Geometry: final body of the model. Coordinates: model frame, mm. Round coordinates to 2 decimals unless told otherwise and drop trailing zeros. Loops run counter-clockwise (first coordinate to the right, second up) from the corner with the lowest first, then second, coordinate; pieces in that order, holes last. Notation, with made-up numbers: M 41,-34 L 90,-34 A18 ccw 90,-30 Z; hole C 85.5,-13.75 d1. An arc over 180 degrees is marked long. Write each question's results on one line, items separated by ' | '.
```python
from build123d import *

# Parameters (mm, degrees)
EXTRUDE_1_DEPTH   = 2
HOLE_WIZARD_M81_D = 9
CHAMFER_1_SIZE    = 2.5


with BuildPart() as part:
    # Эскиз3 → Бобышка-Вытянуть1 (new body)
    with BuildSketch(Plane(origin=(0, 0, 0), x_dir=(1, 0, 0), z_dir=(0, 0, -1))):
        Polygon((0, 0), (100, 0), (100, 75.031110223), (87.059047745, 123.327401537), (0, 100), align=None)
    extrude(amount=EXTRUDE_1_DEPTH)

    # Отверстие с зазором M81 (through all)
    with Locations(Plane(origin=(0, 0, -2), x_dir=(1, 0, 0), z_dir=(0, 0, -1))):
        with Locations((75, 25), (24.776246401, 80.756870704), (69.381378215, 92.708779752), (25, 25)):
            Hole(HOLE_WIZARD_M81_D / 2)

    # Фаска1
    chamfer_1_edges = [part.edges().sort_by_distance(p)[0] for p in [
        (87.059047745, -123.327401537, -1),
        (100, 0, -1),
        (0, 0, -1),
    ]]
    chamfer(chamfer_1_edges, length=CHAMFER_1_SIZE)


solid = part.part
```
1. Pin query (flat end, axial travel): P1, Ø7, axis at x = 24.78, y = -80.76, coming from the -Z side. Return the tip coordinate at first contact, or that it passes through.
Answer key:
P1: passes through
2. Section B-B (x = 26). Output: boundary loops of the cut face in (y, z), then the cut area to 3 significant figures.
Answer key:
outline: M -106.97,-2 L -85.09,-2 L -85.09,0 L -106.97,0 Z; M -76.43,-2 L -29.39,-2 L -29.39,0 L -76.43,0 Z; M -20.61,-2 L 0,-2 L 0,0 L -20.61,0 Z | area: 179 mm²
3. Section C-C (y = -83.5). Output: boundary loops of the cut face in (x, z), then the cut area to 3 significant figures.
Answer key:
outline: M 0,-2 L 21.21,-2 L 21.21,0 L 0,0 Z; M 28.34,-2 L 97.73,-2 L 97.73,0 L 28.34,0 Z | area: 181 mm²
4. Section D-D (z = -0.35). Output: boundary loops of the cut face in (x, y).
Answer key:
outline: M 0,-100 L 84.64,-122.68 L 87.71,-120.91 L 100,-75.03 L 100,-2.5 L 97.5,0 L 2.5,0 L 0,-2.5 Z; hole C 24.78,-80.76 d9; hole C 25,-25 d9; hole C 69.38,-92.71 d9; hole C 75,-25 d9
5. Section A-A (y = -25). Output: boundary loops of the cut face in (x, z).
Answer key:
outline: M 0,-2 L 20.5,-2 L 20.5,0 L 0,0 Z; M 29.5,-2 L 70.5,-2 L 70.5,0 L 29.5,0 Z; M 79.5,-2 L 100,-2 L 100,0 L 79.5,0 Z
6. Draft query along X for faces 1 (the face through (49, -62, 0)), 2 (the face through (1.2, -1.3, -1)), 3 (the face through (25.36, -85.22, -0.99)), 4 (the face through (72.581, -28.794, -0.986)). Return one class per face: pulls with the +X half, pulls with the -X half, needs draft (parallel to the pull), parting line crosses it, or undercut.
Answer key:
face 1: needs draft | face 2: pulls with the -X half | face 3: undercut | face 4: undercut
7. Ray query, probe 1 along X at (y, z) = (-25, -1.4); probe 2 along Y at (x, z) = (25, -0.9); probe 3 along Y at (x, z) = (75, -1.1). Return the intervals inside material, ascending.
Answer key:
probe 1: x = 0 to 20.5, 29.5 to 70.5, 79.5 to 100 | probe 2: y = -106.7 to -85.25, -76.26 to -29.5, -20.5 to 0 | probe 3: y = -120.1 to -29.5, -20.5 to 0
